Read the model definition and answer for the solid it produces. Units are mm, in the model's axes. Coordinates: 2 decimals unless noted, no trailing zeros. Loops run counter-clockwise (first coordinate to the right, second up) from the corner with the lowest first, then second, coordinate; pieces in that order, holes last. Notation, with made-up numbers: (47, 6.5) - (60, 6.5) arc R19 cw to (60, 15.5) - close; hole circle Ø4 at (30.25, -11). An arc over 180 degrees is marked (long way). One line per question, with ' | ' between items. Start each with the question number.
Autodesk Inventor part; units mm, degrees
ref_plane "YZ Plane" through (0, 0, 0) normal (1, 0, 0) x (0, 1, 0)
ref_plane "XZ Plane" through (0, 0, 0) normal (0, 1, 0) x (-1, 0, 0)
ref_plane "XY Plane" through (0, 0, 0) normal (0, 0, 1) x (1, 0, 0)
sketch "スケッチ1" plane through (0, 0, 0) normal (0, 0, 1) x (1, 0, 0)
  circle A0 centre (0, 0) radius 67.5
  dimension "d0" = 135
extrude "プレート1" add sketch "スケッチ1" along normal blind 2
sketch "スケッチ2" plane through (0, 0, 2) normal (0, 0, 1) x (1, 0, 0)
  circle A0 centre (0, 0) radius 38.5
  dimension "d2" = 77
extrude "押し出し1" cut sketch "スケッチ2" against normal through all
sketch "スケッチ3" plane through (0, 0, 2) normal (0, 0, 1) x (1, 0, 0)
  circle A0 centre (0, 0) radius 62.5
  point P0 (16.1762, 60.3704)
  point P1 (-16.1762, 60.3704)
  point P2 (-44.1942, 44.1942)
  point P3 (-60.3704, 16.1762)
  point P4 (-60.3704, -16.1762)
  point P5 (-44.1942, -44.1942)
  point P6 (-16.1762, -60.3704)
  point P7 (16.1762, -60.3704)
  point P8 (44.1942, -44.1942)
  point P9 (60.3704, -16.1762)
  point P10 (60.3704, 16.1762)
  point P11 (44.1942, 44.1942)
  dimension "d5" = 125
  dimension "d8" = 360
  dimension "d36" = 0
hole "穴1" at (16.1762, 60.3704, 2) at (-16.1762, 60.3704, 2) at (-44.1942, 44.1942, 2) at (-60.3704, 16.1762, 2) at (-60.3704, -16.1762, 2) at (-44.1942, -44.1942, 2) at (-16.1762, -60.3704, 2) at (16.1762, -60.3704, 2) at (44.1942, -44.1942, 2) at (60.3704, -16.1762, 2) at (60.3704, 16.1762, 2) at (44.1942, 44.1942, 2) direction (0, 0, -1) diameter 4.3 end through all
sketch "スケッチ4" plane through (0, 0, 2) normal (0, 0, 1) x (1, 0, 0)
  circle A0 centre (0, 0) radius 49
  point P0 (-34.6482, 34.6482)
  point P1 (-34.6482, -34.6482)
  point P2 (34.6482, -34.6482)
  point P3 (34.6482, 34.6482)
  dimension "d17" = 98
  dimension "d20" = 360
  dimension "d29" = 0
hole "穴2" at (-34.6482, 34.6482, 2) at (-34.6482, -34.6482, 2) at (34.6482, -34.6482, 2) at (34.6482, 34.6482, 2) direction (0, 0, -1) diameter 4.3 end through all
sketch "スケッチ6" plane through (0, 0, 0) normal (0, 0, -1) x (-1, 0, 0)
  circle A0 centre (0, 0) radius 37.5
  line L0 (-4.75, -42.3) -> (4.75, -42.3)
  line L1 (-4.75, -37.5) -> (4.75, -37.5)
  circle A1 centre (0, -37.5) radius 4.8
  point P0 (-4.75, -51.1)
  point P1 (4.75, -51.1)
  dimension "d37" = 75
  dimension "d38" = 9.5
  dimension "d39" = 8.8
  dimension "d40" = 13.6
  dimension "d41" = 4.75
hole "穴3" at (4.75, -51.1, 0) at (-4.75, -51.1, 0) direction (0, 0, 1) diameter 2.2 end through all
equation "\"d15\" = Thickness"
equation "\"d27\" = Thickness"
equation "\"d47\" = Thickness"
equation "\"d1\" = Thickness"
equation "\"BendRadius\" = Thickness"
equation "\"BendReliefWidth\" = Thickness"
equation "\"BendReliefDepth\" = 0.5 * Thickness"
equation "\"CornerReliefSize\" = 4 * Thickness"
equation "\"MinimumRemnant\" = 2 * Thickness"
equation "\"TransitionRadius\" = BendRadius"
equation "\"JacobiRadiusSize\" = BendRadius"
equation "\"GapSize\" = Thickness"
properties part number "unit-j2-plate1" material "CFRP"
1) The mould has two halves that part along X. Classify faces 1 (the flat face through (29, -29, 2)), 2 (the cylindrical face through (35.472, -36.634, 0.986)), 3 (the cylindrical face through (-53.57, 41.07, 0.99)): released by +X, released by -X, zero draft, split by the parting line, or undercut.
2) The part is cut by section A-A on y = 0. Write down the section's boundary in (x, z), and give its area (3 significant figures).
3) Given pin 1 Ø1.5 at (x, y) = (48.5, 47) entering from -Z; pin 2 Ø3.5 at (x, y) = (-16.18, 60.37) entering from -Z; pin 3 Ø1 at (x, z) = (-19.5, 0.5) entering from -Y, each flat-ended and moving along its own axis, determine where each tip first touches the part or whether it passes through.
4) Find the intervals of material crossed by line 1 along X through (y, z) = (-14.5, 0.3); line 2 along X through (y, z) = (27, 1.75); line 3 along X through (y, z) = (29, 1.15), in increasing order. Write a range as from..to.
5) The part is cut by section C-C on z = 0.6. Count the separate pieces of the cut face and the enclosed holes in it, and give its area (3 significant figures).
Answer below:
1) face 1: zero draft | face 2: undercut | face 3: split by the parting line
2) outline: (-67.5, 0) - (-38.5, 0) - (-38.5, 2) - (-67.5, 2) - close; (38.5, 0) - (67.5, 0) - (67.5, 2) - (38.5, 2) - close | area: 116 mm2
3) pin 1: z = 0 | pin 2: through | pin 3: y = -64.77
4) line 1: -65.92..-61.72, -59.02..-35.67, 35.67..59.02, 61.72..65.92 | line 2: -61.86..-27.45, 27.45..61.86 | line 3: -60.95..-25.32, 25.32..60.95
5) separate pieces: 1 | enclosed holes: 19 | area: 9,420 mm2
